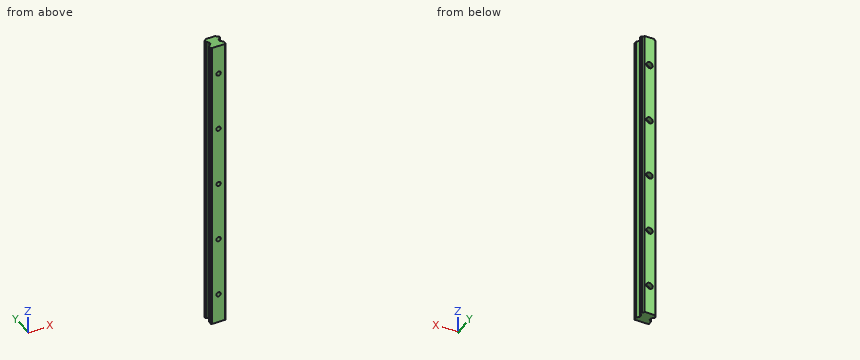
from build123d import *

# Parameters (mm, degrees)
EXTRUDE_1_DEPTH     = 300
SKETCH_2_R          = 3.25
CUT_EXTRUDE_1_DEPTH = 5.3
SKETCH_3_R          = 2.25
CUT_EXTRUDE_2_DEPTH = 301.250462115


with BuildPart() as part:
    # Model → Бобышка-Вытянуть1 (new body)
    with BuildSketch(Plane.XY):
        with BuildLine():
            Line((6.8, 0), (7.5, 0.7))
            Line((7.5, 0.7), (7.5, 3.6994391))
            Line((7.5, 3.6994391), (4.7998047, 6.3996344))
            Line((4.7998047, 6.3996344), (4.7998047, 8.409149262))
            Line((4.7998047, 8.409149262), (5.20075838, 8.810103152))
            ThreePointArc((5.20075838, 8.810103152), (5.668922208, 9.789261508), (6.648080611, 10.257425237))
            Line((6.648080611, 10.257425237), (7.5, 11.109345046))
            Line((7.5, 11.109345046), (7.5, 12.449454443))
            Line((7.5, 12.449454443), (6.634490912, 13.314965186))
            ThreePointArc((6.634490912, 13.314965186), (5.668922174, 13.781617126), (5.202270193, 14.747185846))
            Line((5.202270193, 14.747185846), (4.949456226, 15))
            Line((4.949456226, 15), (-4.949456226, 15))
            Line((-4.949456226, 15), (-5.202270193, 14.747185846))
            ThreePointArc((-5.202270193, 14.747185846), (-5.668922174, 13.781617126), (-6.634490912, 13.314965186))
            Line((-6.634490912, 13.314965186), (-7.5, 12.449454443))
            Line((-7.5, 12.449454443), (-7.5, 11.109345046))
            Line((-7.5, 11.109345046), (-6.648080611, 10.257425238))
            ThreePointArc((-6.648080611, 10.257425238), (-5.668922208, 9.789261508), (-5.20075838, 8.810103152))
            Line((-5.20075838, 8.810103152), (-4.7998047, 8.409149262))
            Line((-4.7998047, 8.409149262), (-4.7998047, 6.3996344))
            Line((-4.7998047, 6.3996344), (-7.5, 3.6994391))
            Line((-7.5, 3.6994391), (-7.5, 0.7))
            Line((-7.5, 0.7), (-6.8, 0))
            Line((-6.8, 0), (6.8, 0))
        make_face()
    extrude(amount=EXTRUDE_1_DEPTH)

    # Эскиз2 → Вырез-Вытянуть1 (cut)
    with BuildSketch(Plane(origin=(0, 15, 0), x_dir=(1, 0, 0), z_dir=(0, 1, 0))):
        with Locations(Location((0, -30, 0), (0, 0, 180))):
            Circle(SKETCH_2_R)
        with Locations(Location((0, -90, 0), (0, 0, 180))):
            Circle(SKETCH_2_R)
        with Locations(Location((0, -150, 0), (0, 0, 180))):
            Circle(SKETCH_2_R)
        with Locations(Location((0, -210, 0), (0, 0, 180))):
            Circle(SKETCH_2_R)
        with Locations(Location((0, -270, 0), (0, 0, 180))):
            Circle(SKETCH_2_R)
        with Locations((0, -330)):
            Circle(SKETCH_2_R)
        with Locations((0, -390)):
            Circle(SKETCH_2_R)
        with Locations((0, -450)):
            Circle(SKETCH_2_R)
        with Locations((0, -510)):
            Circle(SKETCH_2_R)
        with Locations((0, -570)):
            Circle(SKETCH_2_R)
    extrude(amount=-CUT_EXTRUDE_1_DEPTH, mode=Mode.SUBTRACT)

    # Эскиз3 → Вырез-Вытянуть2 (cut, through all)
    with BuildSketch(Plane(origin=(0, 9.7, 0), x_dir=(1, 0, 0), z_dir=(0, 1, 0))):
        with Locations(Location((0, -30, 0), (0, 0, 180))):
            Circle(SKETCH_3_R)
        with Locations(Location((0, -90, 0), (0, 0, 180))):
            Circle(SKETCH_3_R)
        with Locations(Location((0, -150, 0), (0, 0, 180))):
            Circle(SKETCH_3_R)
        with Locations(Location((0, -210, 0), (0, 0, 180))):
            Circle(SKETCH_3_R)
        with Locations(Location((0, -270, 0), (0, 0, 180))):
            Circle(SKETCH_3_R)
        with Locations((0, -330)):
            Circle(SKETCH_3_R)
        with Locations((0, -390)):
            Circle(SKETCH_3_R)
        with Locations((0, -450)):
            Circle(SKETCH_3_R)
        with Locations((0, -510)):
            Circle(SKETCH_3_R)
        with Locations((0, -570)):
            Circle(SKETCH_3_R)
    extrude(amount=-CUT_EXTRUDE_2_DEPTH, mode=Mode.SUBTRACT)


solid = part.part
The listing builds one solid part. Answer for the finished solid, in the listing's coordinates (mm). Round coordinates to 2 decimals unless told otherwise and drop trailing zeros. Write each loop counter-clockwise with the first axis right and the second up, starting at its lowest first coordinate (ties: lowest second). Pieces come first, ordered by that corner, then holes. Notation, with made-up numbers: (77.5, -22.75) - (91.5, -22.75) arc R25 ccw to (91.5, 12.25) - close; hole circle Ø10 at (-6.5, 53.5). An arc over 180 degrees is marked (long way). Use one line per item in the form item = value. Start each with the question number.
Item 1: A cutting plane is placed at A-A (z = 241.5). Write down the section's boundary in (x, y), plus the area to 3 significant figures.
Item 2: Flat-ended cylindrical pins translate along their axes: pin 1 Ø2 at (y, z) = (5.5, 155) entering from +X; pin 2 Ø1.6 at (y, z) = (7.5, 201.5) entering from -X; pin 3 Ø4 at (x, z) = (0, 30) entering from -Y; pin 4 Ø5 at (x, z) = (0, 210) entering from +Y. Find the tip coordinate at first contact, or state that the pin passes through.
Item 3: Find the intervals of material crossed by line 1 (Z direction, x = 0, y = 4.5); line 2 (Z direction, x = 0, y = 11.1); line 3 (X direction, y = 12.5, z = 150), in increasing order. Write a range as [from, to].
Item 4: A cutting plane is placed at B-B (x = 0). Give the number of separate pieces and of enclosed holes in the cut face, plus the area to 3 significant figures.
The answers:
q1.outline = (-7.5, 0.7) - (-6.8, 0) - (6.8, 0) - (7.5, 0.7) - (7.5, 3.7) - (4.8, 6.4) - (4.8, 8.41) - (5.2, 8.81) arc R1.63 cw to (6.65, 10.26) - (7.5, 11.11) - (7.5, 12.45) - (6.63, 13.31) arc R1.63 cw to (5.2, 14.75) - (4.95, 15) - (-4.95, 15) - (-5.2, 14.75) arc R1.63 cw to (-6.63, 13.31) - (-7.5, 12.45) - (-7.5, 11.11) - (-6.65, 10.26) arc R1.63 cw to (-5.2, 8.81) - (-4.8, 8.41) - (-4.8, 6.4) - (-7.5, 3.7) - close
q1.area = 191 mm^2
q2.pin_1 = 6.7
q2.pin_2 = -4.8
q2.pin_3 = through
q2.pin_4 = 9.7
q3.line_1 = [0, 27.75], [32.25, 87.75], [92.25, 147.75], [152.25, 207.75], [212.25, 267.75], [272.25, 300]
q3.line_2 = [0, 26.75], [33.25, 86.75], [93.25, 146.75], [153.25, 206.75], [213.25, 266.75], [273.25, 300]
q3.line_3 = [-7.45, -3.25], [3.25, 7.45]
q4.separate_pieces = 6
q4.enclosed_holes = 0
q4.area = 4,110 mm^2
